Check sheet for the modelled part. Datum: model origin and axes. Units: mm. A direction names the side the tool comes from. Round coordinates to 2 decimals unless told otherwise and drop trailing zeros. Write each loop counter-clockwise with the first axis right and the second up, starting at its lowest first coordinate (ties: lowest second). Pieces come first, ordered by that corner, then holes.
Item 1: Section check C-C, the plane y = -11. Record the cut outline in (x, z).
Item 2: Section check B-B, the plane z = -72.5. Record the cut outline in (x, y), plus the area to 3 significant figures.
Item 3: Material ranges on line 1 along Z through (x, y) = (2, 23); line 2 along X through (y, z) = (23, -99); line 3 along X through (y, z) = (-7.5, -121), recorded low to high.
Item 4: Section check A-A, the plane x = 0. Record the cut outline in (y, z), plus the area to 3 significant figures.
Item 5: Depth check by flat-ended pin: pin 1 (6 mm diameter, centred on x = -2.5, y = 22.5, fed in from -Z); pin 2 (3 mm diameter, centred on y = 22.5, z = -33, fed in from -X); pin 3 (2 mm diameter, centred on y = 6.5, z = -80.5, fed in from +X); pin 4 (6 mm diameter, centred on y = 21.5, z = -54, fed in from +X). Enter the tip coordinate at first touch or a pass-through.
Item 6: Set-up check for faces 1 (the flat face through (5, 22, -46)), 2 (the flat face through (0, 3, 10)), 3 (the flat face through (-5, 22, -46)): record each of +Z, -Z, +X, -X, +Y, -Y from which the full face is reachable in a straight line by a thin tool's end or side.
from build123d import *

# Parameters (mm, degrees)
EXTRUDE1_DEPTH      = 10
EXTRUDE1_DEPTH_BACK = 150
CUT_EXTRUDE1_DEPTH  = 50


with BuildPart() as part:
    # Sketch1 → Extrude1 (new, two sides: drawn at the far end of the back side and taken through both)
    with BuildSketch(Plane.XY.offset(-EXTRUDE1_DEPTH_BACK)):
        with BuildLine():
            Line((-5, 25), (-5, 19.364916731))
            ThreePointArc((-5, 19.364916731), (0, -20), (5, 19.364916731))
            Line((5, 19.364916731), (5, 25))
            Line((5, 25), (-5, 25))
        make_face()
    extrude(amount=EXTRUDE1_DEPTH + EXTRUDE1_DEPTH_BACK)

    # Sketch2 → Cut-Extrude1 (cut)
    with BuildSketch(Plane(origin=(0, 0, -150), x_dir=(-1, 0, 0), z_dir=(0, 0, -1))):
        with BuildLine():
            Line((-5, 19.364916731), (-5, 25))
            Line((-5, 25), (5, 25))
            Line((5, 25), (5, 19.364916731))
            ThreePointArc((5, 19.364916731), (0, 20), (-5, 19.364916731))
        make_face()
    extrude(amount=-CUT_EXTRUDE1_DEPTH, mode=Mode.SUBTRACT)


solid = part.part
Values found:
1. outline: (-16.7, -150) - (16.7, -150) - (16.7, 10) - (-16.7, 10) - close
2. outline: (-5, 19.36) arc R20 ccw (long way) to (5, 19.36) - (5, 25) - (-5, 25) - close
2. area: 1,310 mm2
3. line 1: z = -100 to 10
3. line 2: x = -5 to 5
3. line 3: x = -18.54 to 18.54
4. outline: (-20, -150) - (20, -150) - (20, -100) - (25, -100) - (25, 10) - (-20, 10) - close
4. area: 6,950 mm2
5. pin 1: stops at z = -150
5. pin 2: stops at x = -5
5. pin 3: stops at x = 19.23
5. pin 4: stops at x = 7.6
6. face 1: +Z, -Z, +X, +Y
6. face 2: +Z, +X, -X, +Y, -Y
6. face 3: +Z, -Z, -X, +Y
